The model under review builds one solid part; all positions refer to its coordinate system, in mm. Round coordinates to 2 decimals unless told otherwise and drop trailing zeros. Loops run counter-clockwise (first coordinate to the right, second up) from the corner with the lowest first, then second, coordinate; pieces in that order, holes last. Notation, with made-up numbers: M 77,29.25 L 122,29.25 A14 cw 122,36.25 Z; hole C 36,-2 d4. An arc over 180 degrees is marked long. Return JSON: item names as keys, results as strings. Group by question number.
Q1. To check wall thickness, follow line 1 along Y through (x, z) = (-0.5, 4); line 2 along X through (y, z) = (-10, 1); line 3 along Y through (x, z) = (-8.5, 0.5). State the ranges of each line that lie inside material, in increasing order.
Q2. Clearance check with flat-ended pins moving along their axes: pin 1 Ø1.5 at (x, z) = (-8.5, 2) entering from -Y; pin 2 Ø5 at (x, z) = (12.5, 1.5) entering from +Y; pin 3 Ø1 at (y, z) = (16.5, 7) entering from -X. State where each tip first meets the part, or that it passes through.
Q3. Draft analysis for pull direction Y (two halves, no side actions). For faces 1 (the face through (-16.058, 0.707, 5.914)), 2 (the face through (-16.058, -0.707, 2.976)), 3 (the face through (-18.897, 14.49, 4.785)), 4 (the face through (-9, 17, 0)), state which applies: pulls with the +Y half, pulls with the -Y half, needs draft (parallel to the pull), parting line crosses it, or undercut.
Q4. Consider section C-C (z = 8). State the section outline as (x, y) points (1 decimal), and give its area (3 significant figures).
Autodesk Inventor part; units mm, degrees
ref_plane "YZ Plane" through (0, 0, 0) normal (1, 0, 0) x (0, 1, 0)
ref_plane "XZ Plane" through (0, 0, 0) normal (0, 1, 0) x (-1, 0, 0)
ref_plane "XY Plane" through (0, 0, 0) normal (0, 0, 1) x (1, 0, 0)
sketch "Sketch1" plane through (0, 0, 0) normal (0, 0, 1) x (1, 0, 0)
  circle A0 centre (0, 0) radius 15.875
  circle A1 centre (0, 0) radius 23.8125
  dimension "d0" = 31.75
  dimension "d1" = 47.625
extrude "Extrusion1" add sketch "Sketch1" along normal blind 8.89
chamfer "Chamfer1" distance 0.7937 angle 45 1 edges at (-23.8125, 0, 0)
chamfer "Chamfer2" distance 3.175 angle 45 2 edges at (-15.875, 0, 8.89) (-15.875, 0, 0)
properties part number "Tire" material "Rubber, Silicone"
Values:
{
 "1": {"line 1": "y = -23.81 to -15.87, 15.87 to 23.81", "line 2": "x = -21.61 to -15.03, 15.03 to 21.61", "line 3": "y = -21.93 to -16.49, 16.49 to 21.93"},
 "2": {"pin 1": "stops at y = -22.52", "pin 2": "stops at y = 21.61", "pin 3": "stops at x = -17.64"},
 "3": {"face 1": "undercut", "face 2": "undercut", "face 3": "parting line crosses it", "face 4": "needs draft"},
 "4": {"outline": "C 0,0 d47.6; hole C 0,0 d36.3", "area": "745 mm2"}
}
